Work out the finished part from the listing and answer in its coordinate system (mm). A direction names the side the tool comes from. Give positions to 0.01 mm unless a question says otherwise; leave off trailing zeros. Loops run counter-clockwise (first coordinate to the right, second up) from the corner with the lowest first, then second, coordinate; pieces in that order, holes last. Notation, with made-up numbers: M 67.25,80.25 L 97.25,80.25 A19 ccw 97.25,95.25 Z; hole C 27.5,49 d6. An arc over 180 degrees is marked long. Use a Markdown table: item, result.
```python
from build123d import *

# Parameters (mm, degrees)
F0_R     = 7.9957240037
F1_DEPTH = 15


# Not quite as in the source:
# - a feature names something its author has since deleted; it is built from what else it names


with BuildPart() as f1:
    # F0 (on Top) → F1 (new body)
    with BuildSketch(Plane.XY):
        with BuildLine():
            Line((60.2735915523, 0), (-31.5768626855, 0))
            ThreePointArc((-31.5768626855, 0), (-45.7189983092, -5.8578643763), (-51.5768626855, -20))
            Line((-51.5768626855, -20), (-51.5768626855, -40))
            Line((-51.5768626855, -40), (-31.5768626855, -40))
            Line((-31.5768626855, -40), (-31.5768626855, -10))
            Line((-31.5768626855, -10), (-22.5768626855, -10))
            Line((-22.5768626855, -10), (-22.5768626855, -40))
            Line((-22.5768626855, -40), (83.3676023199, -40))
            Line((83.3676023199, -40), (83.3676023199, -20))
            Line((83.3676023199, -20), (83.3676023199, 0))
            Line((83.3676023199, 0), (60.2735915523, 0))
        make_face()
        with BuildLine():
            Line((131.1026292389, 122.6794919243), (60.2735915523, 0))
            Line((60.2735915523, 0), (83.3676023199, 0))
            Line((83.3676023199, 0), (83.3676023199, -20))
            Line((83.3676023199, -20), (83.3676023199, -40))
            Line((83.3676023199, -40), (165.7436453902, 102.6794919243))
            ThreePointArc((165.7436453902, 102.6794919243), (167.7416538403, 117.8558728264), (158.4231373145, 130))
            ThreePointArc((158.4231373145, 130), (143.2467564125, 131.9980084501), (131.1026292389, 122.6794919243))
        make_face()
        with Locations((148.4231373145, 112.6794919243)):
            Circle(F0_R, mode=Mode.SUBTRACT)
    extrude(amount=F1_DEPTH)


solid = f1.part
```
(1) The mould has two halves that part along Y. Classify faces 3 (the flat face through (15, 0, 7)), 4 (the cylindrical face through (152.113, 105.586, 7.395)), 5 (the flat face through (123.98, 30.34, 7.4)): released by +Y, released by -Y, zero draft, split by the parting line, or undercut.
Entries:
| item | result |
|---|---|
| face 3 | released by +Y |
| face 4 | undercut |
| face 5 | released by -Y |
(2) Consider probe 1 along Y at (x, z) = (0.5, 10.5); probe 2 along X at (y, z) = (111.5, 2.75); probe 3 along X at (y, z) = (65.5, 4). Determine where each line is inside the solid, lowest interval first. Write a range as [from, to].
Entries:
| item | result |
|---|---|
| probe 1 | y = [-40, 0] |
| probe 2 | x = [124.65, 140.51], [156.33, 168.39] |
| probe 3 | x = [98.09, 144.28] |
(3) A cutting plane is placed at C-C (z = 8.5). Write down the section's boundary in (x, y).
Entries:
| item | result |
|---|---|
| outline | M -51.58,-40 L -31.58,-40 L -31.58,-10 L -22.58,-10 L -22.58,-40 L 83.37,-40 L 165.74,102.68 A20 ccw 131.1,122.68 L 60.27,0 L -31.58,0 A20 ccw -51.58,-20 Z; hole C 148.42,112.68 d15.99 |
(4) Which of the six approach directions +Z, -Z, +X, -X, +Y, -Y give full straight-line access (tool end or side, diameter ignored) to faces 1 (the flat face through (-31.577, -25, 7)), 2 (the flat face through (-51.577, -30, 7))?
Entries:
| item | result |
|---|---|
| face 1 | +Z, -Z, -Y |
| face 2 | +Z, -Z, -X, +Y, -Y |
(5) A cutting plane is placed at B-B (x = 151). Write down the section's boundary in (y, z).
Entries:
| item | result |
|---|---|
| outline | M 77.14,0 L 105.11,0 L 105.11,15 L 77.14,15 Z; M 120.25,0 L 132.51,0 L 132.51,15 L 120.25,15 Z |
(6) A cutting plane is placed at A-A (y = -15). Write down the section's boundary in (x, z).
Entries:
| item | result |
|---|---|
| outline | M -50.94,0 L -31.58,0 L -31.58,15 L -50.94,15 Z; M -22.58,0 L 97.8,0 L 97.8,15 L -22.58,15 Z |
(7) Given P1, Ø4.5, axis at x = 14, z = 4, coming from the +Y side; P2, Ø8, axis at y = -3, z = 6.5, coming from the +X side; P3, Ø6, axis at x = 106, z = 13, coming from the +Y side, each flat-ended and moving along its own axis, determine where each tip first touches the part or whether it passes through.
Entries:
| item | result |
|---|---|
| P1 | stops at y = 0 |
| P2 | stops at x = 107.04 |
| P3 | stops at y = 84.4 |
(8) A cutting plane is placed at D-D (x = 51). Write down the section's boundary in (y, z), and give its area (3 significant figures).
Entries:
| item | result |
|---|---|
| outline | M -40,0 L 0,0 L 0,15 L -40,15 Z |
| area | 600 mm² |
